The figure shows three views and two pictorial views of one solid part (mm, origin at its lowest corner). Answer the questions. A direction names the side the tool comes from. Give positions to 0.01 mm unless a question says otherwise; leave off trailing zeros. Write each loop counter-clockwise with the first axis right and the second up, starting at its lowest first coordinate (ties: lowest second). Pieces come first, ordered by that corner, then holes. Notation, with made-up numbers: (89, -24) - (116, -24) arc R13 cw to (116, -7) - close; hole circle Ø6 at (-23.75, 47.5). An arc over 180 degrees is marked (long way). Use a Markdown table: item, result. Add a question column.
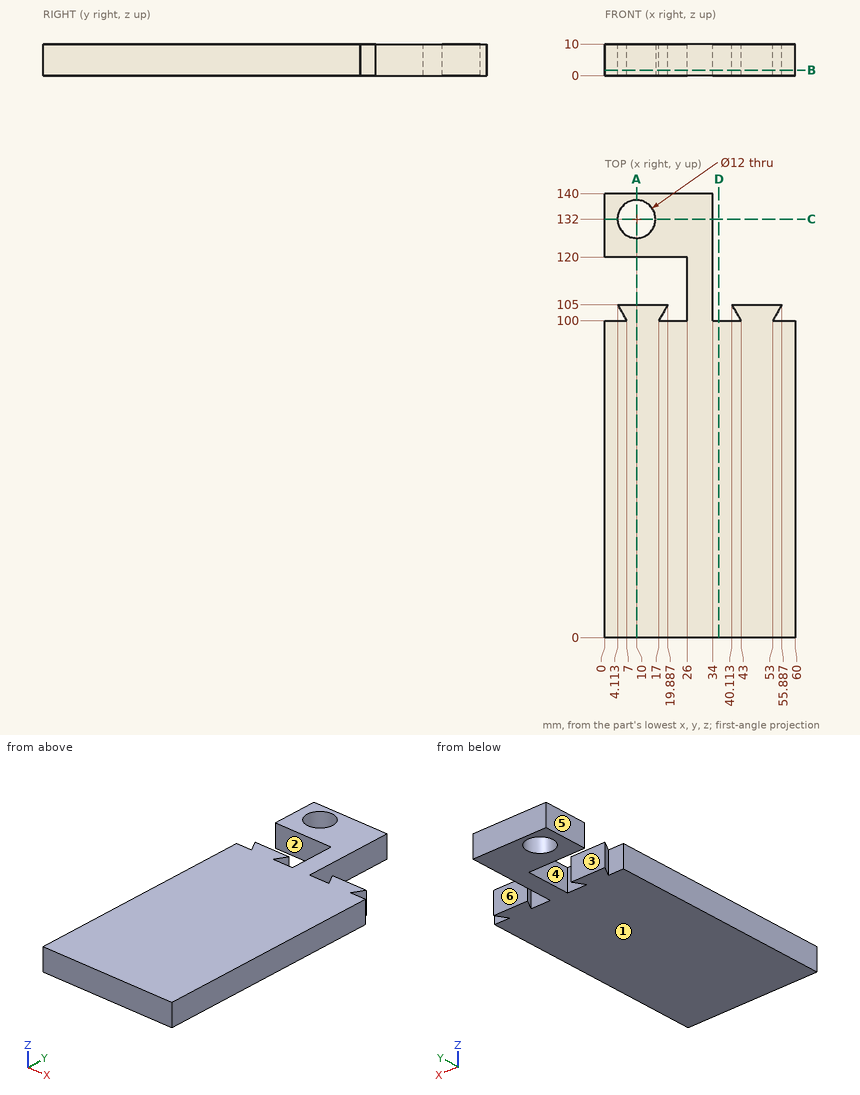
1. The part is cut by section D-D (x = 36). Give the vertices of the cut face in (y, z).
2. Consider L1, parallel to Y at x = 10, z = 4.5; L2, parallel to Y at x = 3.5, z = 6; L3, parallel to Y at x = 14.5, z = 6.25. Determine where each line is inside the solid, lowest interval first. Write a range as [from, to].
3. Given P1, Ø2.5, axis at x = 40.5, z = 7.5, coming from the +Y side; P2, Ø1.5, axis at y = 102, z = 2.5, coming from the -X side; P3, Ø9.5, axis at x = 10, y = 132, coming from the -Z side, each flat-ended and moving along its own axis, determine where each tip first touches the part or whether it passes through.
4. The part is cut by section B-B (z = 1.75). Give the vertices of the cut face in (x, y), and give its area (3 significant figures).
5. The part is cut by section C-C (y = 132). Give the vertices of the cut face in (x, z).
6. For a pull along Y with two mould halves and no side action, classify the marked faces 3, 4, 5 and 6 as released by +Y, released by -Y, zero draft, split by the parting line, or undercut.
7. The part is cut by section A-A (x = 10). Give the vertices of the cut face in (y, z).
8. Which of the six approach directions +Z, -Z, +X, -X, +Y, -Y give full straight-line access (tool end or side, diameter ignored) to the marked faces 1 and 2?
Check values:
| question | item | result |
|---|---|---|
| 1 | outline | (0, 0) - (100, 0) - (100, 10) - (0, 10) - close |
| 2 | L1 | y = [0, 105], [120, 126], [138, 140] |
| 2 | L2 | y = [0, 100], [120, 140] |
| 2 | L3 | y = [0, 105], [120, 128.03], [135.97, 140] |
| 3 | P1 | stops at y = 105 |
| 3 | P2 | stops at x = 5.41 |
| 3 | P3 | passes through |
| 4 | outline | (0, 0) - (60, 0) - (60, 100) - (53, 100) - (55.89, 105) - (40.11, 105) - (43, 100) - (34, 100) - (34, 140) - (0, 140) - (0, 120) - (26, 120) - (26, 100) - (17, 100) - (19.89, 105) - (4.11, 105) - (7, 100) - (0, 100) - close; hole circle Ø12 at (10, 132) |
| 4 | area | 6,860 mm2 |
| 5 | outline | (0, 0) - (4, 0) - (4, 10) - (0, 10) - close; (16, 0) - (34, 0) - (34, 10) - (16, 10) - close |
| 6 | face 3 | undercut |
| 6 | face 4 | undercut |
| 6 | face 5 | zero draft |
| 6 | face 6 | released by +Y |
| 7 | outline | (0, 0) - (105, 0) - (105, 10) - (0, 10) - close; (120, 0) - (126, 0) - (126, 10) - (120, 10) - close; (138, 0) - (140, 0) - (140, 10) - (138, 10) - close |
| 8 | face 1 | -Z, +X, -X, +Y, -Y |
| 8 | face 2 | +Z, -Z, -X |
